```python
from build123d import *

# Parameters (mm, degrees)
F0_W     = 150
F0_H     = 40
F1_DEPTH = 5
F2_R     = 2
F3_DEPTH = 25
F4_R     = 2
F5_DEPTH = 25
F6_W     = 40.1
F6_H     = 40
F7_DEPTH = 2
F8_R     = 0.25


with BuildPart() as f1:
    # F0 (on Top) → F1 (new body)
    with BuildSketch(Plane.XY):
        with Locations((75, 20)):
            Rectangle(F0_W, F0_H)
    extrude(amount=F1_DEPTH)

    # F2 (on face) → F3 (cut)
    with BuildSketch(Plane.XY.offset(5)):
        with Locations((6.25, 34)):
            Circle(F2_R)
        with Locations((6.25, 6)):
            Circle(F2_R)
        with Locations((143.75, 34)):
            Circle(F2_R)
        with Locations((143.75, 6)):
            Circle(F2_R)
    extrude(amount=-F3_DEPTH, mode=Mode.SUBTRACT)

    # F4 (on face) → F5 (cut)
    with BuildSketch(Plane.XY.offset(5)):
        with Locations((70, 35)):
            Circle(F4_R)
        with Locations((70, 5)):
            Circle(F4_R)
        with Locations((100, 35)):
            Circle(F4_R)
        with Locations((100, 5)):
            Circle(F4_R)
    extrude(amount=-F5_DEPTH, mode=Mode.SUBTRACT)

    # F6 (on face) → F7 (cut)
    with BuildSketch(Plane.XY.offset(5)):
        with Locations((85, 20)):
            Rectangle(F6_W, F6_H)
    extrude(amount=-F7_DEPTH, mode=Mode.SUBTRACT)

    # F8
    f8_edges = [f1.edges().sort_by_distance(p)[0] for p in [
        (64.95, 20, 5),
        (64.95, 20, 3),
        (105.05, 20, 5),
        (105.05, 20, 3),
    ]]
    fillet(f8_edges, radius=F8_R)


solid = f1.part
```
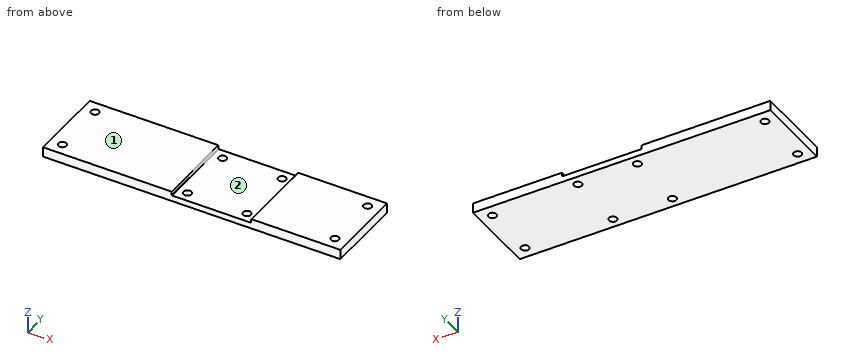
Here's how the part is built. I have some questions about the finished solid (model axes, mm). Face numbers are marked on the shaded views. Round coordinates to 2 decimals unless told otherwise and drop trailing zeros. Order: outer loops, then holes, each group sorted by start corner. A loop starts at its lowest first (then second) coordinate and runs counter-clockwise, first axis right, second up. Notation, with made-up numbers: (44, 46) -> (77, 46) arc R21 cw to (77, 71) -> close; hole circle Ø2 at (28.5, 85). An arc over 180 degrees is marked (long way). Use a Markdown table: item, result. Add a question column.
(1) If we mould it in two halves opening along X, with no side actions, what happens to the marked faces 1 and 2? For each: released by +X, released by -X, zero draft, split by the parting line, or undercut.
(2) Suppose I cut it at A-A, the plane x = 70. Please give me the cut outline in (y, z), and give its area (3 significant figures).
(3) For pin 1 Ø3 at (x, y) = (143.75, 6) entering from +Z; pin 2 Ø10 at (x, y) = (78.5, 25.5) entering from +Z, each with a flat end and sliding along its axis, tell me the tip position at first contact or that it passes through.
(4) Suppose I cut it at C-C, the plane y = 9.5. Please give me the cut outline in (x, z).
(5) Suppose I cut it at B-B, the plane z = 1.2. Count the separate pieces of the cut face and the enclosed holes in it, and give its area (3 significant figures).
(6) Suppose I cut it at D-D, the plane x = 6.25. Please give me the cut outline in (y, z).
(7) I need wall thicknesses on line 1 along Y through (x, z) = (70, 2.2); line 2 along Y through (x, z) = (143.75, 2); line 3 along X through (y, z) = (2.5, 3.65). Which ranges of each line are inside material? Lowest first, please.
Verdict:
| question | item | result |
|---|---|---|
| 1 | face 1 | zero draft |
| 1 | face 2 | undercut |
| 2 | outline | (0, 0) -> (3, 0) -> (3, 3) -> (0, 3) -> close; (7, 0) -> (33, 0) -> (33, 3) -> (7, 3) -> close; (37, 0) -> (40, 0) -> (40, 3) -> (37, 3) -> close |
| 2 | area | 96.0 mm2 |
| 3 | pin 1 | through |
| 3 | pin 2 | z = 3 |
| 4 | outline | (0, 0) -> (150, 0) -> (150, 5) -> (105.3, 5) arc R0.25 ccw to (105.05, 4.75) -> (105.05, 3.25) arc R0.25 cw to (104.8, 3) -> (65.2, 3) arc R0.25 cw to (64.95, 3.25) -> (64.95, 4.75) arc R0.25 ccw to (64.7, 5) -> (0, 5) -> close |
| 5 | separate pieces | 1 |
| 5 | enclosed holes | 8 |
| 5 | area | 5,900 mm2 |
| 6 | outline | (0, 0) -> (4, 0) -> (4, 5) -> (0, 5) -> close; (8, 0) -> (32, 0) -> (32, 5) -> (8, 5) -> close; (36, 0) -> (40, 0) -> (40, 5) -> (36, 5) -> close |
| 7 | line 1 | 0 to 3, 7 to 33, 37 to 40 |
| 7 | line 2 | 0 to 4, 8 to 32, 36 to 40 |
| 7 | line 3 | 0 to 64.95, 105.05 to 150 |
